Source: CAD feature listing. Evaluate the final solid. Frame: model axes, mm. Face numbers are marked on the shaded views. A direction names the side the tool comes from. Coordinates: 2 decimals unless noted, no trailing zeros. Write each loop counter-clockwise with the first axis right and the second up, starting at its lowest first coordinate (ties: lowest second). Pieces come first, ordered by that corner, then holes. Notation, with made-up numbers: M -16.75,70.25 L 11.25,70.25 A28 cw 11.25,96.25 Z; hole C 28.25,-14.5 d1. An arc over 180 degrees is marked long. One line per item, written item: value. Start each with the question number.
Item 1: Cut plane C-C, the plane z = 15.5. Output: boundary loops of the cut face in (x, y).
Item 2: Pin query (flat end, axial travel): P1, Ø2, axis at y = -2.5, z = -3, coming from the +X side; P2, Ø4.5, axis at x = 15.5, z = -15.5, coming from the -Y side; P3, Ø2.5, axis at x = 15.5, z = 15.5, coming from the +Y side. Return the tip coordinate at first contact, or that it passes through.
Item 3: Cut plane B-B, the plane y = 7. Output: boundary loops of the cut face in (x, z).
Item 4: Ray query, L1, parallel to Z at x = -15.5, y = 23.5; L2, parallel to Z at x = 15, y = 27. Return the intervals inside material, ascending. Write a range as from..to.
Item 5: Cut plane D-D, the plane z = 0. Output: boundary loops of the cut face in (x, y).
Item 6: Set-up query: the marked faces 1 and 2. Return all of +Z, -Z, +X, -X, +Y, -Y with unobstructed straight access to the full face (end or side cutting, diameter ignored); none if empty.
Item 7: Cut plane A-A, the plane x = 15.5. Output: boundary loops of the cut face in (y, z), then the cut area to 3 significant figures.
```python
from build123d import *

# Parameters (mm, degrees)
F0_R     = 2.5
F3_DEPTH = 24
F1_R     = 11
F4_DEPTH = 2
F5_DEPTH = 39
F7_D     = 4


with BuildPart() as f3:
    # F0 (on Front) → F3 (new body)
    with BuildSketch(Plane.XZ):
        Circle(F0_R)
    extrude(amount=F3_DEPTH)

    # F1 (on Front) → F4 (join)
    with BuildSketch(Plane.XZ):
        Circle(F1_R)
    extrude(amount=F4_DEPTH)

    # F2 (on Front) → F5 (join)
    with BuildSketch(Plane.XZ):
        Polygon((21, 16.5), (16.5, 21), (-16.5, 21), (-21, 16.5), (-21, -16.5), (-16.5, -21), (16.5, -21), (21, -16.5), align=None)
    extrude(amount=-F5_DEPTH)

    # F7 (through all)
    with Locations(Plane.XZ):
        with Locations((-15.5, 15.5), (15.5, 15.5), (15.5, -15.5), (-15.5, -15.5)):
            Hole(F7_D / 2)


solid = f3.part
```
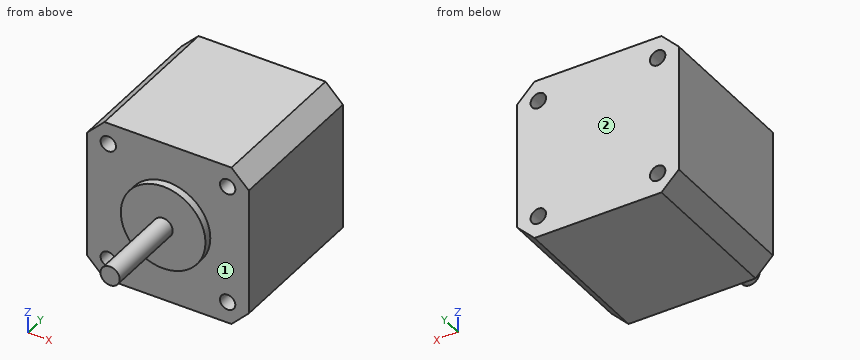
From the geometry:
1. outline: M -21,0 L -17.5,0 L -17.5,39 L -21,39 Z; M -13.5,0 L 13.5,0 L 13.5,39 L -13.5,39 Z; M 17.5,0 L 21,0 L 21,39 L 17.5,39 Z
2. P1: stops at x = 10.79
2. P2: stops at y = 0
2. P3: passes through
3. outline: M -21,-16.5 L -16.5,-21 L 16.5,-21 L 21,-16.5 L 21,16.5 L 16.5,21 L -16.5,21 L -21,16.5 Z; hole C -15.5,-15.5 d4; hole C -15.5,15.5 d4; hole C 15.5,-15.5 d4; hole C 15.5,15.5 d4
4. L1: z = -21..-17.5, -13.5..13.5, 17.5..21
4. L2: z = -21..-17.44, -13.56..13.56, 17.44..21
5. outline: M -21,0 L -11,0 L -11,-2 L -2.5,-2 L -2.5,-24 L 2.5,-24 L 2.5,-2 L 11,-2 L 11,0 L 21,0 L 21,39 L -21,39 Z
6. face 1: -Y
6. face 2: +Z, -Z, +X, -X, +Y
7. outline: M 0,-21 L 39,-21 L 39,-17.5 L 0,-17.5 Z; M 0,-13.5 L 39,-13.5 L 39,13.5 L 0,13.5 Z; M 0,17.5 L 39,17.5 L 39,21 L 0,21 Z
7. area: 1,330 mm²
